from build123d import *

# Parameters (mm, degrees)
SKETCH1_W              = 254
SKETCH1_H              = 88.9
BOSS_EXTRUDE1_DEPTH    = 6
F_10_CLEARANCE_HOLE1_D = 6.0452
SKETCH4_R              = 11.2
SKETCH4_R_2            = 1.65
CUT_EXTRUDE1_DEPTH     = 135.687796403


with BuildPart() as part:
    # Sketch1 → Boss-Extrude1 (new body)
    with BuildSketch(Plane.YZ):
        Rectangle(SKETCH1_W, SKETCH1_H)
    extrude(amount=-BOSS_EXTRUDE1_DEPTH)

    # #10 Clearance Hole1 (through all)
    with Locations(Plane.YZ):
        with Locations((118.2625, 38.1), (-118.2625, 38.1), (-118.2625, -38.1), (118.2625, -38.1)):
            Hole(F_10_CLEARANCE_HOLE1_D / 2)

    # Sketch4 → Cut-Extrude1 (cut, through all)
    with BuildSketch(Plane.YZ):
        with Locations(Location((0, 0, 0), (0, 0, 270))):
            Circle(SKETCH4_R)
        with Locations(Location((-15.5, 15.5, 0), (0, 0, 270))):
            Circle(SKETCH4_R_2)
        with Locations(Location((15.5, 15.5, 0), (0, 0, 90))):
            Circle(SKETCH4_R_2)
        with Locations(Location((15.5, -15.5, 0), (0, 0, 270))):
            Circle(SKETCH4_R_2)
        with Locations(Location((-15.5, -15.5, 0), (0, 0, 90))):
            Circle(SKETCH4_R_2)
        with Locations(Location((75, 0, 0), (0, 0, 270))):
            Circle(SKETCH4_R)
        with Locations(Location((59.5, 15.5, 0), (0, 0, 270))):
            Circle(SKETCH4_R_2)
        with Locations(Location((90.5, 15.5, 0), (0, 0, 90))):
            Circle(SKETCH4_R_2)
        with Locations(Location((90.5, -15.5, 0), (0, 0, 270))):
            Circle(SKETCH4_R_2)
        with Locations(Location((59.5, -15.5, 0), (0, 0, 90))):
            Circle(SKETCH4_R_2)
        with Locations(Location((-75, 0, 0), (0, 0, 270))):
            Circle(SKETCH4_R)
        with Locations(Location((-90.5, -15.5, 0), (0, 0, 90))):
            Circle(SKETCH4_R_2)
        with Locations(Location((-59.5, -15.5, 0), (0, 0, 270))):
            Circle(SKETCH4_R_2)
        with Locations(Location((-59.5, 15.5, 0), (0, 0, 90))):
            Circle(SKETCH4_R_2)
        with Locations(Location((-90.5, 15.5, 0), (0, 0, 270))):
            Circle(SKETCH4_R_2)
    extrude(amount=-CUT_EXTRUDE1_DEPTH, mode=Mode.SUBTRACT)


solid = part.part
For this review, take the finished solid that the model builds, in its own axes (mm). Give positions to 0.01 mm unless a question says otherwise; leave off trailing zeros. Loops run counter-clockwise (first coordinate to the right, second up) from the corner with the lowest first, then second, coordinate; pieces in that order, holes last. Notation, with made-up numbers: M 1,-7.5 L 26,-7.5 A24 ccw 26,2.5 Z; hole C -4.75,69.5 d5. An arc over 180 degrees is marked long. Answer as a JSON object with one key per item and string values. Group by question number.
Q1. For probe 1 along Z at (x, y) = (-1.35, -90.5); probe 2 along Y at (x, z) = (-3, -0.5); probe 3 along Z at (x, y) = (-2.1, -117), list the stretches that pass through material, from the lowest coordinate up. Write a range as [from, to].
Q2. Add section A-A on z = -38.1. Give the boundary of the cut face in (x, y), and give its area (3 significant figures).
Q3. Add section B-B on y = 75. Give the boundary of the cut face in (x, z).
Q4. Mouldability with a two-part tool opening along Y and no side actions: class faces 1 (the flat face through (0, -2, 20)), 2 (the cylindrical face through (-3.04, -117.61, -41.05)), 3 (the flat face through (-3, 127, -1)), 4 (the cylindrical face through (-3.04, 120.66, 36.26)) as +Y half, -Y half, draft (parallel to the pull), parting line (faces both ways), or undercut.
Q5. Add section C-C on x = -2.75. Give the number of separate pieces and of enclosed holes in the cut face, and give its area (3 significant figures).
Q6. Add section D-D on y = -77.5. Give the boundary of the cut face in (x, z).
Checked values:
{
 "1": {"probe 1": "[-44.45, -17.15], [-13.85, 13.85], [17.15, 44.45]", "probe 2": "[-127, -86.19], [-63.81, -11.19], [11.19, 63.81], [86.19, 127]", "probe 3": "[-44.45, -40.85], [-35.35, 35.35], [40.85, 44.45]"},
 "2": {"outline": "M -6,-127 L 0,-127 L 0,-121.29 L -6,-121.29 Z; M -6,-115.24 L 0,-115.24 L 0,115.24 L -6,115.24 Z; M -6,121.29 L 0,121.29 L 0,127 L -6,127 Z", "area": "1,450 mm²"},
 "3": {"outline": "M -6,-44.45 L 0,-44.45 L 0,-11.2 L -6,-11.2 Z; M -6,11.2 L 0,11.2 L 0,44.45 L -6,44.45 Z"},
 "4": {"face 1": "draft", "face 2": "undercut", "face 3": "+Y half", "face 4": "undercut"},
 "5": {"separate pieces": "1", "enclosed holes": "19", "area": "21,200 mm²"},
 "6": {"outline": "M -6,-44.45 L 0,-44.45 L 0,-10.92 L -6,-10.92 Z; M -6,10.92 L 0,10.92 L 0,44.45 L -6,44.45 Z"}
}
